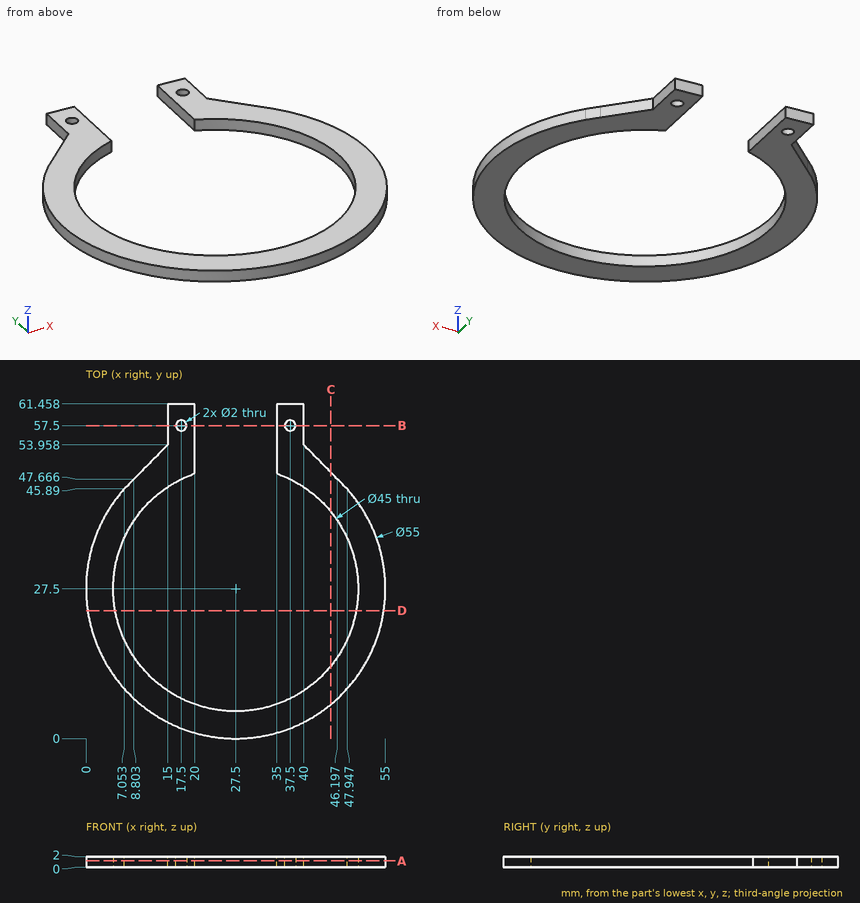
Geometry check sheet. Reference: drawing and pictorial views, mm from the part's lowest x, y, z. Give positions to 0.01 mm unless a question says otherwise; leave off trailing zeros. Order: outer loops, then holes, each group sorted by start corner. A loop starts at its lowest first (then second) coordinate and runs counter-clockwise, first axis right, second up. Notation, with made-up numbers: M -9,-19 L 30,-19 A15 ccw 30,9 Z; hole C 83.25,53.5 d7. An arc over 180 degrees is marked long. Answer in a Markdown table with one row per item. Add a question column.
Q1. Sectioned sample at D-D, the plane y = 23.5. Record the boundary of the cut face in (x, z).
Q2. Sectioned sample at A-A, the plane z = 1.2. Record the boundary of the cut face in (x, y).
Q3. Sectioned sample at B-B, the plane y = 57.5. Record the boundary of the cut face in (x, z), and give its area (3 significant figures).
Q4. Sectioned sample at C-C, the plane x = 45. Record the boundary of the cut face in (y, z).
Q5. Thickness scan on L1, parallel to X at y = 57.5, z = 1.15; L2, parallel to Y at x = 17.5, z = 0.85 (1 decimal); L3, parallel to X at y = 27.5, z = 1.4. Record the ranges inside material, lowest first.
Q6. Gauge pin test, flat ends, axial feed: pin 1 Ø0.6 at (y, z) = (59, 1) entering from -X; pin 2 Ø1 at (x, z) = (48.5, 1.5) entering from -Y. Record the tip position at first contact, or that the pin passes through.
Verdict:
| question | item | result |
|---|---|---|
| 1 | outline | M 0.29,0 L 5.36,0 L 5.36,2 L 0.29,2 Z; M 49.64,0 L 54.71,0 L 54.71,2 L 49.64,2 Z |
| 2 | outline | M 7.05,45.89 A27.5 ccw long 47.95,45.89 L 40,53.96 L 40,61.46 L 35,61.46 L 35,48.71 A22.5 cw long 20,48.71 L 20,61.46 L 15,61.46 L 15,53.96 Z; hole C 17.5,57.5 d2; hole C 37.5,57.5 d2 |
| 3 | outline | M 15,0 L 16.5,0 L 16.5,2 L 15,2 Z; M 18.5,0 L 20,0 L 20,2 L 18.5,2 Z; M 35,0 L 36.5,0 L 36.5,2 L 35,2 Z; M 38.5,0 L 40,0 L 40,2 L 38.5,2 Z |
| 3 | area | 12.0 mm² |
| 4 | outline | M 6.29,0 L 13.36,0 L 13.36,2 L 6.29,2 Z; M 41.64,0 L 48.88,0 L 48.88,2 L 41.64,2 Z |
| 5 | L1 | 15 to 16.5, 18.5 to 20, 35 to 36.5, 38.5 to 40 |
| 5 | L2 | 1.9 to 7.3, 47.7 to 56.5, 58.5 to 61.5 |
| 5 | L3 | 0 to 5, 50 to 55 |
| 6 | pin 1 | x = 15 |
| 6 | pin 2 | y = 9.17 |
